from build123d import *

# Parameters (mm, degrees)
SKIZZE1_R                        = 33
AUFSATZ_LINEAR_AUSTRAGEN1_DEPTH  = 3
F_3_2_3_2_DURCHMESSER_BOHRUNG1_D = 3.2


with BuildPart() as part:
    # Skizze1 → Aufsatz-Linear austragen1 (new body)
    with BuildSketch(Plane.XY):
        with BuildLine():
            Line((-38.5, -19.150718002), (-38.5, 19.150718002))
            ThreePointArc((-38.5, 19.150718002), (0, 43), (38.5, 19.150718002))
            Line((38.5, 19.150718002), (38.5, -19.150718002))
            ThreePointArc((38.5, -19.150718002), (0, -43), (-38.5, -19.150718002))
        make_face()
        Circle(SKIZZE1_R, mode=Mode.SUBTRACT)
    extrude(amount=AUFSATZ_LINEAR_AUSTRAGEN1_DEPTH)

    # Ø3.2 (3.2) Durchmesser Bohrung1 (through all)
    with Locations(Plane.XY.offset(3)):
        with Locations((-34.347488991, 20.5), (0, 40), (0, -40), (34.347488991, -20.5), (34.347488991, 20.5), (-34.347488991, -20.5)):
            Hole(F_3_2_3_2_DURCHMESSER_BOHRUNG1_D / 2)


solid = part.part
CAD build for the part. Positions are in the model's coordinates, mm. Round coordinates to 2 decimals unless told otherwise and drop trailing zeros. Write each loop counter-clockwise with the first axis right and the second up, starting at its lowest first coordinate (ties: lowest second). Pieces come first, ordered by that corner, then holes. Notation, with made-up numbers: M 66,61.25 L 80,61.25 A13 cw 80,81.25 Z; hole C 70,-29 d3. An arc over 180 degrees is marked long. Put each result on its own line as item: value. Start each with the question number.
1) Drill centre lines: probe 1 along X at (y, z) = (-20, 2.45); probe 2 along Y at (x, z) = (-1, 1.95); probe 3 along Y at (x, z) = (24, 1). Where is each one in solid material? Low to high. Write a range as [from, to].
2) Pull direction Y, two halves, no side cores. Call faces 1 (the cylindrical face through (-0.74, 38.58, 1.48)), 2 (the cylindrical face through (0.668, -42.995, 1.479)), 3 (the flat face through (-8.4, 32.1, 0)): pulls with the +Y half, pulls with the -Y half, needs draft (parallel to the pull), parting line crosses it, or undercut.
3) Pin check, flat tips, straight feed: pin 1 Ø5 at (x, y) = (0, 40) entering from -Z; pin 2 Ø1.5 at (y, z) = (-31.5, 1.5) entering from -X. Stop position of each tip, or through.
4) Saw through at A-A, the plane y = 0. Write the cut outline in (x, z).
5) Saw through at D-D, the plane y = 20.5. Write the cut outline in (x, z), and give its area (3 significant figures).
6) Saw through at C-C, the plane z = 2. Write the cut outline in (x, y), and give its area (3 significant figures).
7) Saw through at B-B, the plane x = 0. Write the cut outline in (y, z), and give its area (3 significant figures).
Resolved:
1. probe 1: [-38.07, -35.87], [-32.83, -26.25], [26.25, 32.83], [35.87, 38.07]
1. probe 2: [-42.99, -41.25], [-38.75, -32.98], [32.98, 38.75], [41.25, 42.99]
1. probe 3: [-35.68, -22.65], [22.65, 35.68]
2. face 1: undercut
2. face 2: pulls with the -Y half
2. face 3: needs draft
3. pin 1: z = 0
3. pin 2: x = -30.06
4. outline: M -38.5,0 L -33,0 L -33,3 L -38.5,3 Z; M 33,0 L 38.5,0 L 38.5,3 L 33,3 Z
5. outline: M -37.8,0 L -35.95,0 L -35.95,3 L -37.8,3 Z; M -32.75,0 L -25.86,0 L -25.86,3 L -32.75,3 Z; M 25.86,0 L 32.75,0 L 32.75,3 L 25.86,3 Z; M 35.95,0 L 37.8,0 L 37.8,3 L 35.95,3 Z
5. area: 52.4 mm²
6. outline: M -38.5,-19.15 A43 ccw 38.5,-19.15 L 38.5,19.15 A43 ccw -38.5,19.15 Z; hole C -34.35,-20.5 d3.2; hole C -34.35,20.5 d3.2; hole C 0,0 d66; hole C 0,-40 d3.2; hole C 0,40 d3.2; hole C 34.35,-20.5 d3.2; hole C 34.35,20.5 d3.2
6. area: 2,110 mm²
7. outline: M -43,0 L -41.6,0 L -41.6,3 L -43,3 Z; M -38.4,0 L -33,0 L -33,3 L -38.4,3 Z; M 33,0 L 38.4,0 L 38.4,3 L 33,3 Z; M 41.6,0 L 43,0 L 43,3 L 41.6,3 Z
7. area: 40.8 mm²
